from build123d import *

# Parameters (mm, degrees)
EXTRUDE_1_DEPTH     = 20
SKETCH_2_R          = 3
CUT_EXTRUDE_1_DEPTH = 39
SKETCH_4_W          = 3
SKETCH_4_H          = 20
CUT_EXTRUDE_3_DEPTH = 8
SKETCH_5_W          = 35
SKETCH_5_H          = 20
CUT_EXTRUDE_4_DEPTH = 1
SKETCH_6_W          = 20
SKETCH_6_H          = 28
CUT_EXTRUDE_5_DEPTH = 1
SKETCH_8_W          = 20
SKETCH_8_H          = 2
CUT_EXTRUDE_6_DEPTH = 18
EXTRUDE_2_DEPTH     = 10
SKETCH_10_R         = 1.5
CUT_EXTRUDE_7_DEPTH = 10


with BuildPart() as part:
    # 草图1 → 凸台-拉伸1 (new body)
    with BuildSketch(Plane.XY):
        Polygon((0, 0), (0, 38), (3, 38), (3, 3), (38, 3), (38, 0), align=None)
    extrude(amount=EXTRUDE_1_DEPTH)

    # 草图2 → 切除-拉伸1 (cut, through all)
    with BuildSketch(Plane.ZY):
        with Locations((5, 16)):
            Circle(SKETCH_2_R)
    extrude(amount=-CUT_EXTRUDE_1_DEPTH, mode=Mode.SUBTRACT)

    # 草图4 → 切除-拉伸3 (cut)
    with BuildSketch(Plane(origin=(0, 38, 0), x_dir=(1, 0, 0), z_dir=(0, 1, 0))):
        with Locations((1.5, -10)):
            Rectangle(SKETCH_4_W, SKETCH_4_H)
    extrude(amount=-CUT_EXTRUDE_3_DEPTH, mode=Mode.SUBTRACT)

    # 草图5 → 切除-拉伸4 (cut)
    with BuildSketch(Plane(origin=(0, 3, 0), x_dir=(1, 0, 0), z_dir=(0, 1, 0))):
        with Locations((20.5, -10)):
            Rectangle(SKETCH_5_W, SKETCH_5_H)
    extrude(amount=-CUT_EXTRUDE_4_DEPTH, mode=Mode.SUBTRACT)

    # 草图6 → 切除-拉伸5 (cut)
    with BuildSketch(Plane(origin=(3, 0, 0), x_dir=(0, 0, -1), z_dir=(1, 0, 0))):
        with Locations((-10, 16)):
            Rectangle(SKETCH_6_W, SKETCH_6_H)
    extrude(amount=-CUT_EXTRUDE_5_DEPTH, mode=Mode.SUBTRACT)

    # 草图8 → 切除-拉伸6 (cut)
    with BuildSketch(Plane(origin=(38, 0, 0), x_dir=(0, 0, -1), z_dir=(1, 0, 0))):
        with Locations((-10, 1)):
            Rectangle(SKETCH_8_W, SKETCH_8_H)
    extrude(amount=-CUT_EXTRUDE_6_DEPTH, mode=Mode.SUBTRACT)

    # 草图9 → 凸台-拉伸2 (add)
    with BuildSketch(Plane(origin=(0, 0, 0), x_dir=(-1, 0, 0), z_dir=(0, 0, -1))):
        Polygon((0, 0), (0, 30), (-2, 30), (-2, 2), (-20, 2), (-20, 0), align=None)
    extrude(amount=EXTRUDE_2_DEPTH)

    # 草图10 → 切除-拉伸7 (cut)
    with BuildSketch(Plane(origin=(0, 2, 0), x_dir=(1, 0, 0), z_dir=(0, 1, 0))):
        with Locations((16, -15)):
            Circle(SKETCH_10_R)
        with Locations((16, 5)):
            Circle(SKETCH_10_R)
        with Locations((6, -15)):
            Circle(SKETCH_10_R)
        with Locations((6, 5)):
            Circle(SKETCH_10_R)
    extrude(amount=-CUT_EXTRUDE_7_DEPTH, mode=Mode.SUBTRACT)


solid = part.part
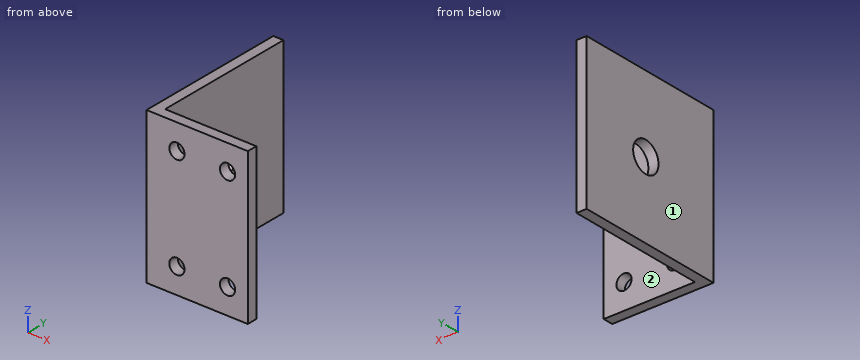
Input: part model. Units: mm. Frame: model coordinates. Face numbers are marked on the shaded views. A direction names the side the tool comes from. Give positions to 0.01 mm unless a question says otherwise; leave off trailing zeros. Order: outer loops, then holes, each group sorted by start corner. A loop starts at its lowest first (then second) coordinate and runs counter-clockwise, first axis right, second up. Notation, with made-up numbers: M 23,12 L 65,12 A21 cw 65,24 Z; hole C 76,32.25 d2. An arc over 180 degrees is marked long. Answer as a JSON object with one key per item and string values.
1. Reachability of the marked faces 1 and 2 from +Z, -Z, +X, -X, +Y, -Y: full face, straight path, thin tool, end or side. Return the list, or none.
Result sheet:
{"face 1": "+Z, -Z, -X, +Y, -Y", "face 2": "+Z, -Z, +X, +Y"}
2. Cut plane D-D, the plane z = 15. Output: boundary loops of the cut face in (x, y), and give its area (3 significant figures).
Result sheet:
{"outline": "M 0,0 L 4.5,0 L 4.5,2 L 2,2 L 2,30 L 0,30 Z; M 7.5,0 L 14.5,0 L 14.5,2 L 7.5,2 Z; M 17.5,0 L 20,0 L 20,2 L 17.5,2 Z", "area": "84.0 mm²"}
3. First-contact query: P1, Ø4, axis at x = 16, z = 15, coming from the +Y side; P2, Ø8.5, axis at y = 15, z = 7, coming from the +X side. Flat tips, straight axial feed; report the tip coordinate or a pass-through.
Result sheet:
{"P1": "y = 2", "P2": "x = 2"}
4. Cut plane B-B, the plane y = 16. Output: boundary loops of the cut face in (x, z), and give its area (3 significant figures).
Result sheet:
{"outline": "M 0,-10 L 2,-10 L 2,2 L 0,2 Z; M 0,8 L 2,8 L 2,20 L 0,20 Z", "area": "48.0 mm²"}
5. Cut plane C-C, the plane x = 16. Output: boundary loops of the cut face in (y, z), and give its area (3 significant figures).
Result sheet:
{"outline": "M 0,-10 L 2,-10 L 2,-6.5 L 0,-6.5 Z; M 0,-3.5 L 2,-3.5 L 2,13.5 L 0,13.5 Z; M 0,16.5 L 2,16.5 L 2,20 L 0,20 Z", "area": "48.0 mm²"}
6. Cut plane A-A, the plane z = 5. Output: boundary loops of the cut face in (x, y), and give its area (3 significant figures).
Result sheet:
{"outline": "M 0,0 L 20,0 L 20,2 L 2,2 L 2,13 L 0,13 Z; M 0,19 L 2,19 L 2,30 L 0,30 Z", "area": "84.0 mm²"}
7. Ray query, line 1 (Z direction, x = 16, y = 0.95); line 2 (X direction, y = 0.5, z = -5); line 3 (Y direction, x = 0.5, z = 5). Return the intervals inside material, ascending. Write a range as [from, to].
Result sheet:
{"line 1": "[-10, -6.5], [-3.5, 13.5], [16.5, 20]", "line 2": "[0, 4.5], [7.5, 14.5], [17.5, 20]", "line 3": "[0, 13], [19, 30]"}
